Read the model definition and answer for the solid it produces. Units are mm, in the model's axes. A direction names the side the tool comes from. Give positions to 0.01 mm unless a question says otherwise; leave off trailing zeros. Order: outer loops, then holes, each group sorted by start corner. A loop starts at its lowest first (then second) coordinate and runs counter-clockwise, first axis right, second up. Notation, with made-up numbers: (63.25, 51) - (88.25, 51) arc R5 ccw to (88.25, 58) - close; hole circle Ø5 at (40.5, 33). An arc over 180 degrees is marked (long way). Write item = value, one per line.
```python
from build123d import *

# Parameters (mm, degrees)
BOSS_EXTRUDE1_DEPTH = 17.5
CUT_EXTRUDE1_DEPTH  = 15.5
SKETCH7_W           = 23.8
SKETCH7_H           = 23.8
CUT_EXTRUDE4_DEPTH  = 37.949289574
SKETCH7_5_W         = 25
SKETCH7_5_H         = 4.2
SKETCH7_5_R         = 1
BOSS_EXTRUDE3_DEPTH = 4
FILLET2_R           = 1.5
CUT_EXTRUDE6_REACH  = 46.612
SKETCH14_W          = 11
SKETCH14_H          = 2.5
SKETCH20_W          = 11
SKETCH20_H          = 2.5
CUT_EXTRUDE7_DEPTH  = 45.612218057
SKETCH21_W          = 24
SKETCH21_H          = 17.1
SKETCH21_H_2        = 3.6
BOSS_EXTRUDE4_DEPTH = 0.5
CHAMFER2_SIZE       = 0.5
CUT_EXTRUDE8_DEPTH  = 1
CUT_EXTRUDE9_REACH  = 57.057
FILLET3_R           = 1


# Some blends are built 0.0001 mm under size
with BuildPart() as part:
    # Sketch1 → Boss-Extrude1 (new body)
    with BuildSketch(Plane(origin=(0, 0, 0), x_dir=(1, 0, 0), z_dir=(0, 1, 0))):
        Polygon((-15, 20), (15, 20), (15, -20), (15, -30), (-15, -30), (-15, -20), align=None)
    extrude(amount=BOSS_EXTRUDE1_DEPTH)

    # Sketch2 → Cut-Extrude1 (cut)
    with BuildSketch(Plane(origin=(0, 17.5, 0), x_dir=(1, 0, 0), z_dir=(0, 1, 0))):
        Polygon((-13, 18), (13, 18), (13, -18), (13, -28), (-13, -28), (-13, -18), align=None)
    extrude(amount=-CUT_EXTRUDE1_DEPTH, mode=Mode.SUBTRACT)

    # Sketch7 → Cut-Extrude4 (cut, through all)
    with BuildSketch(Plane(origin=(0, 2, 0), x_dir=(1, 0, 0), z_dir=(0, 1, 0))):
        with Locations((0, 1.5)):
            Rectangle(SKETCH7_W, SKETCH7_H)
    extrude(amount=-CUT_EXTRUDE4_DEPTH, mode=Mode.SUBTRACT)

    # Sketch7<5> → Boss-Extrude3 (add)
    # profile 1 of 2: a face of its own
    with BuildSketch(Plane(origin=(0, 2, 0), x_dir=(1, 0, 0), z_dir=(0, 1, 0))):
        with Locations((0, 15.9)):
            Rectangle(SKETCH7_5_W, SKETCH7_5_H)
        with Locations(Location((0, 15.903889524, 0), (0, 0, 270))):
            Circle(SKETCH7_5_R, mode=Mode.SUBTRACT)
    # profile 2 of 2: a face of its own
    with BuildSketch(Plane(origin=(0, 2, 0), x_dir=(1, 0, 0), z_dir=(0, 1, 0))):
        Polygon((-11.9, -10.4), (-12.5, -10.4), (-12.5, -14.45), (0, -14.45), (12.5, -14.45), (12.5, -10.4), align=None)
        with Locations(Location((0, -11.95, 0), (0, 0, 90))):
            Circle(SKETCH7_5_R, mode=Mode.SUBTRACT)
    extrude(amount=BOSS_EXTRUDE3_DEPTH)

    # Fillet2
    fillet2_edges = [part.edges().sort_by_distance(p)[0] for p in [
        (15, 8.75, 30),
        (-15, 8.75, 30),
        (-15, 8.75, -20),
        (15, 8.75, -20),
        (0, 0, 30),
        (-15, 0, 5),
        (0, 0, -20),
        (15, 0, 5),
    ]]
    fillet(fillet2_edges, radius=FILLET2_R)

    # Sketch14 → Cut-Extrude6 (cut, up to next)
    with BuildSketch(Plane(origin=(-13, 0, 0), x_dir=(0, 0, -1), z_dir=(1, 0, 0)), mode=Mode.PRIVATE) as cut_extrude6_sk1:
        with Locations((-17.5, 13.25)):
            Rectangle(SKETCH14_W, SKETCH14_H)
    cut_extrude6_tool1 = extrude(cut_extrude6_sk1.sketch, amount=-CUT_EXTRUDE6_REACH, mode=Mode.PRIVATE) & part.part
    add(cut_extrude6_tool1.solids().sort_by_distance((-13, 13.25, 17.5))[0], mode=Mode.SUBTRACT)

    # Sketch20 → Cut-Extrude7 (cut, through all)
    with BuildSketch(Plane.ZY.offset(-13)):
        with Locations((-7.698338616, 13.25)):
            Rectangle(SKETCH20_W, SKETCH20_H)
    extrude(amount=-CUT_EXTRUDE7_DEPTH, mode=Mode.SUBTRACT)

    # Sketch21 → Boss-Extrude4 (add)
    with BuildSketch(Plane.XZ):
        with Locations((0, 18.95)):
            Rectangle(SKETCH21_W, SKETCH21_H)
        with Locations((0, -15.2)):
            Rectangle(SKETCH21_W, SKETCH21_H_2)
    extrude(amount=BOSS_EXTRUDE4_DEPTH)

    # Chamfer2
    chamfer2_edges = [part.edges().sort_by_distance(p)[0] for p in [
        (12, -0.5, 18.95),
        (-12, -0.5, 18.95),
        (-12, -0.5, -15.2),
        (0, -0.5, -17),
        (12, -0.5, -15.2),
        (0, -0.5, 27.5),
    ]]
    chamfer(chamfer2_edges, length=CHAMFER2_SIZE - 0.0001)  # a hair under: the kernel refuses the full size

    # Sketch22 → Cut-Extrude8 (cut)
    with BuildSketch(Plane(origin=(0, 17.5, 0), x_dir=(1, 0, 0), z_dir=(0, 1, 0))):
        Polygon((-13, 18), (-14, 18), (-14, -19.085850071), (-14, -29.085850071), (14, -29.085850071), (14, -19.085850071), (14, 18), (13, 18), (13, -28), (-13, -28), align=None)
    extrude(amount=-CUT_EXTRUDE8_DEPTH, mode=Mode.SUBTRACT)

    # Sketch23 → Cut-Extrude9 (cut, up to next)
    with BuildSketch(Plane.XY.offset(30), mode=Mode.PRIVATE) as cut_extrude9_sk1:
        with BuildLine():
            Line((-3, 17.5), (3, 17.5))
            ThreePointArc((3, 17.5), (0, 14.5), (-3, 17.5))
        make_face()
    cut_extrude9_tool1 = extrude(cut_extrude9_sk1.sketch, amount=-CUT_EXTRUDE9_REACH, mode=Mode.PRIVATE) & part.part
    add(cut_extrude9_tool1.solids().sort_by_distance((0, 16.22676, 30))[0], mode=Mode.SUBTRACT)

    # Fillet3
    # the kernel refuses this fillet: 1 mm, written as the material it adds along each edge
    with BuildSketch(Plane(origin=(12.5, 2, -13.8), x_dir=(1, 0, 0), z_dir=(0, 0, -1))) as fillet3_piece_1_section:
        with BuildLine():
            CenterArc((1, -0.866025404), FILLET3_R, 120, 60)
            Line((0, -0.866025404), (0, 0))
            Line((0, 0), (0.5, 0))
        make_face()
    fillet3_piece_1 = extrude(amount=6.365063509, mode=Mode.PRIVATE)
    fillet3_piece_1 = split(fillet3_piece_1, bisect_by=Plane(origin=(12.5, 2, -20), z_dir=(0, 0, 1)), keep=Keep.TOP, mode=Mode.PRIVATE)
    add(fillet3_piece_1)
    with BuildSketch(Plane(origin=(-12.5, 2, -20.165063509), x_dir=(-1, 0, 0), z_dir=(0, 0, 1))) as fillet3_piece_2_section:
        with BuildLine():
            CenterArc((1, -0.866025404), FILLET3_R, 120, 60)
            Line((0, -0.866025404), (0, 0))
            Line((0, 0), (0.5, 0))
        make_face()
    fillet3_piece_2 = extrude(amount=6.365063509, mode=Mode.PRIVATE)
    fillet3_piece_2 = split(fillet3_piece_2, bisect_by=Plane(origin=(-12.5, 2, -20), z_dir=(0, 0, 1)), keep=Keep.TOP, mode=Mode.PRIVATE)
    add(fillet3_piece_2)
    with BuildSketch(Plane(origin=(-12.5, 2, 10.4), x_dir=(-1, 0, 0), z_dir=(0, 0, 1)), Plane(origin=(12.5, 2, 14.45), x_dir=(1, 0, 0), z_dir=(0, 0, -1))) as fillet3_piece_3:
        with BuildLine():
            CenterArc((FILLET3_R, -FILLET3_R), FILLET3_R, 90, 90)
            Line((0, -FILLET3_R), (0, 0))
            Line((0, 0), (FILLET3_R, 0))
        make_face()
    extrude(amount=4.05)
    with BuildSketch(Plane(origin=(-12.5, 2, 14.45), x_dir=(0, 0, 1), z_dir=(1, 0, 0))) as fillet3_piece_4:
        with BuildLine():
            CenterArc((FILLET3_R, -FILLET3_R), FILLET3_R, 90, 90)
            Line((0, -FILLET3_R), (0, 0))
            Line((0, 0), (FILLET3_R, 0))
        make_face()
    extrude(amount=25)
    with BuildSketch(Plane(origin=(-15, 2, 14.45), x_dir=(0, 0, 1), z_dir=(1, 0, 0))) as fillet3_piece_5a_section:
        with BuildLine():
            CenterArc((FILLET3_R, -FILLET3_R), FILLET3_R, 90, 90)
            Line((0, -FILLET3_R), (0, 0))
            Line((0, 0), (FILLET3_R, 0))
        make_face()
    fillet3_piece_5a = extrude(amount=27.5, mode=Mode.PRIVATE)
    fillet3_piece_5a = split(fillet3_piece_5a, bisect_by=Plane(origin=(-13, 2, 14.45), z_dir=(1, 0, 0)), keep=Keep.TOP, mode=Mode.PRIVATE)
    fillet3_piece_5a = split(fillet3_piece_5a, bisect_by=Plane(origin=(-12.5, 2, 14.45), z_dir=(-1, 0, 0)), keep=Keep.TOP, mode=Mode.PRIVATE)
    with BuildSketch(Plane(origin=(-12.5, 2, 10.4), x_dir=(-1, 0, 0), z_dir=(0, 0, 1))) as fillet3_piece_5b_section:
        with BuildLine():
            CenterArc((FILLET3_R, -FILLET3_R), FILLET3_R, 90, 90)
            Line((0, -FILLET3_R), (0, 0))
            Line((0, 0), (FILLET3_R, 0))
        make_face()
    fillet3_piece_5b = extrude(amount=6.55, mode=Mode.PRIVATE)
    fillet3_piece_5b = split(fillet3_piece_5b, bisect_by=Plane(origin=(-13, 2, 10.4), z_dir=(1, 0, 0)), keep=Keep.TOP, mode=Mode.PRIVATE)
    fillet3_piece_5b = split(fillet3_piece_5b, bisect_by=Plane(origin=(-12.5, 2, 14.45), z_dir=(0, 0, 1)), keep=Keep.TOP, mode=Mode.PRIVATE)
    fillet3_piece_5 = fillet3_piece_5a & fillet3_piece_5b
    add(fillet3_piece_5)
    with BuildSketch(Plane(origin=(12.5, 2, 16.95), x_dir=(1, 0, 0), z_dir=(0, 0, -1))) as fillet3_piece_6a_section:
        with BuildLine():
            CenterArc((FILLET3_R, -FILLET3_R), FILLET3_R, 90, 90)
            Line((0, -FILLET3_R), (0, 0))
            Line((0, 0), (FILLET3_R, 0))
        make_face()
    fillet3_piece_6a = extrude(amount=6.55, mode=Mode.PRIVATE)
    fillet3_piece_6a = split(fillet3_piece_6a, bisect_by=Plane(origin=(13, 2, 16.95), z_dir=(-1, 0, 0)), keep=Keep.TOP, mode=Mode.PRIVATE)
    fillet3_piece_6a = split(fillet3_piece_6a, bisect_by=Plane(origin=(12.5, 2, 14.45), z_dir=(0, 0, 1)), keep=Keep.TOP, mode=Mode.PRIVATE)
    with BuildSketch(Plane(origin=(-12.5, 2, 14.45), x_dir=(0, 0, 1), z_dir=(1, 0, 0))) as fillet3_piece_6b_section:
        with BuildLine():
            CenterArc((FILLET3_R, -FILLET3_R), FILLET3_R, 90, 90)
            Line((0, -FILLET3_R), (0, 0))
            Line((0, 0), (FILLET3_R, 0))
        make_face()
    fillet3_piece_6b = extrude(amount=27.5, mode=Mode.PRIVATE)
    fillet3_piece_6b = split(fillet3_piece_6b, bisect_by=Plane(origin=(13, 2, 14.45), z_dir=(-1, 0, 0)), keep=Keep.TOP, mode=Mode.PRIVATE)
    fillet3_piece_6b = split(fillet3_piece_6b, bisect_by=Plane(origin=(12.5, 2, 14.45), z_dir=(1, 0, 0)), keep=Keep.TOP, mode=Mode.PRIVATE)
    fillet3_piece_6 = fillet3_piece_6a & fillet3_piece_6b
    add(fillet3_piece_6)


solid = part.part
```
1. Determine the mould class of faces 4 (the face through (14, 12, -8)), 5 (the face through (14.55, 0.43, 4.67)), 6 (the face through (14, 14.5, -8)), 7 (the face through (14.57, 9.61, 29.55)) for opening direction Z: +Z half, -Z half, draft (parallel to the pull), parting line (faces both ways), or undercut.
Recorded:
face_4 = undercut
face_5 = draft
face_6 = undercut
face_7 = +Z half
2. Flat-ended cylindrical pins translate along their axes: pin 1 (4.5 mm diameter, centred on x = 0.5, z = -15, fed in from +Y); pin 2 (1 mm diameter, centred on x = 9, z = 20, fed in from +Y); pin 3 (5.5 mm diameter, centred on x = 9, z = -1, fed in from +Y); pin 4 (2 mm diameter, centred on x = -3.5, y = 0, fed in from +Z). Find the tip coordinate at first contact, or state that the pin passes through.
Recorded:
pin_1 = 6
pin_2 = 2
pin_3 = through
pin_4 = 29.91
3. Section D-D (z = 1.5) is taken. Determine the outline of the cut face in (x, y).
Recorded:
outline = (-15, 1.5) arc R1.5 ccw to (-13.5, 0) - (-11.9, 0) - (-11.9, 2) - (-13, 2) - (-13, 16.5) - (-14, 16.5) - (-14, 17.5) - (-15, 17.5) - close; (11.9, 0) - (13.5, 0) arc R1.5 ccw to (15, 1.5) - (15, 17.5) - (14, 17.5) - (14, 16.5) - (13, 16.5) - (13, 2) - (11.9, 2) - close
4. For faces 1 (the face through (-0.19, 0.43, 29.55)), 2 (the face through (12.5, 4, 12)), 3 (the face through (-11.9, 1, -1)), determine the directions among +Z, -Z, +X, -X, +Y, -Y from which every point of the face is accessible in a straight line to the end or side of a thin tool.
Recorded:
face_1 = +Z, +X, -X, -Y
face_2 = +Y
face_3 = +Y, -Y
5. Section C-C (z = -12.5) is taken. Determine the outline of the cut face in (x, y).
Recorded:
outline = (-15, 1.5) arc R1.5 ccw to (-13.5, 0) - (-11.9, 0) - (-11.9, 2) - (-13, 2) - (-13, 16.5) - (-14, 16.5) - (-14, 17.5) - (-15, 17.5) - close; (11.9, 0) - (13.5, 0) arc R1.5 ccw to (15, 1.5) - (15, 12) - (13, 12) - (13, 2) - (11.9, 2) - close; (13, 14.5) - (15, 14.5) - (15, 17.5) - (14, 17.5) - (14, 16.5) - (13, 16.5) - close
6. Straight lines are drawn through the part: L1, parallel to X at y = 3.85, z = 11.95; L2, parallel to Z at x = 9.75, y = 12.75; L3, parallel to X at y = 8.25, z = 5. For each, find the intervals that lie inside material, in ascending order. Write a range as [from, to].
Recorded:
L1 = [-15, -13], [-12.5, -1], [1, 12.5], [13, 15]
L2 = [-20, -18], [28, 30]
L3 = [-15, -13], [13, 15]
7. Section A-A (y = 4) is taken. Determine the outline of the cut face in (x, z).
Recorded:
outline = (-15, -18.5) arc R1.5 ccw to (-13.5, -20) - (13.5, -20) arc R1.5 ccw to (15, -18.5) - (15, 28.5) arc R1.5 ccw to (13.5, 30) - (-13.5, 30) arc R1.5 ccw to (-15, 28.5) - close; (-12.5, 10.4) - (12.5, 10.4) - (12.5, 14.45) - (-12.5, 14.45) - close; hole (-13, -18) - (-12.5, -18) - (-12.5, -13.8) - (12.5, -13.8) - (12.5, -18) - (13, -18) - (13, 28) - (-13, 28) - close; hole circle Ø2 at (0, -15.9); hole circle Ø2 at (0, 11.95)
